Work out the finished part from the listing and answer in its coordinate system (mm). A direction names the side the tool comes from. Give positions to 0.01 mm unless a question says otherwise; leave off trailing zeros. Write each loop counter-clockwise with the first axis right and the second up, starting at its lowest first coordinate (ties: lowest second). Pieces come first, ordered by that corner, then holes.
1) A tool of negligible diameter and unlimited length cuts with its end or side. For faces 1 (the face through (-110.6, -411.4, 382.62)), 2 (the face through (-313.79, -222.74, 380.68)), from which of +Z, -Z, +X, -X, +Y, -Y can it reach the whole face along a straight path? Write none if from no direction.
2) Straight lines are drawn through the part: probe 1 along X at (y, z) = (-526, 378.5); probe 2 along Y at (x, z) = (-32, 381.25); probe 3 along Y at (x, z) = (-26, 379.5). For each, find the intervals that lie inside material, in ascending order.
3) Find section B-B (z = 379). Count the separate pieces of the cut face and the enclosed holes in it, plus the area to 3 significant figures.
4) Determine the mould class of faces 3 (the face through (-44.44, -546.24, 380.68)), 4 (the face through (-108, -396, 384.62)) for opening direction X: pulls with the +X half, pulls with the -X half, needs draft (parallel to the pull), parting line crosses it, or undercut.
5) Given pin 1 Ø4.5 at (x, y) = (-269.36, -538.87) entering from -Z, flat-ended and moving along its own axis, determine where the tip first touches the part or whether it passes through.
6) Find section A-A (x = -112.5). Determine the outline of the cut face in (y, z).
```python
from build123d import *

# Parameters (mm, degrees)
SKETCH1_R           = 6
SKETCH1_R_2         = 4.5
SKETCH1_R_3         = 6.5
SKETCH1_R_4         = 3.735
SKETCH1_W           = 48
SKETCH1_H           = 20
SKETCH1_W_2         = 49
BOSS_EXTRUDE1_DEPTH = 8
SKETCH2_R           = 2.5
CUT_EXTRUDE1_DEPTH  = 10
CUT_EXTRUDE2_DEPTH  = 2


with BuildPart() as part:
    # Sketch1 → Boss-Extrude1 (new body)
    with BuildSketch(Plane(origin=(0, 0, 384.620141885), x_dir=(-1, 0, 0), z_dir=(0, 0, -1))):
        with BuildLine():
            Line((-108.789156386, -197.798939869), (-108.789156386, -599.798939869))
            ThreePointArc((-108.789156386, -599.798939869), (-107.617583511, -602.627366994), (-104.789156386, -603.798939869))
            Line((-104.789156386, -603.798939869), (327.210843614, -603.798939869))
            ThreePointArc((327.210843614, -603.798939869), (330.039270738, -602.627366994), (331.210843614, -599.798939869))
            Line((331.210843614, -599.798939869), (331.210843614, -197.798939869))
            ThreePointArc((331.210843614, -197.798939869), (330.039270738, -194.970512745), (327.210843614, -193.798939869))
            Line((327.210843614, -193.798939869), (-104.789156386, -193.798939869))
            ThreePointArc((-104.789156386, -193.798939869), (-107.617583511, -194.970512745), (-108.789156386, -197.798939869))
        make_face()
        with Locations((-95.789156386, -206.798939869)):
            Circle(SKETCH1_R, mode=Mode.SUBTRACT)
        with Locations((-95.789156386, -226.798939869)):
            Circle(SKETCH1_R, mode=Mode.SUBTRACT)
        with Locations((146.210843614, -209.798939869)):
            Circle(SKETCH1_R_2, mode=Mode.SUBTRACT)
        with Locations((76.210843614, -209.798939869)):
            Circle(SKETCH1_R_2, mode=Mode.SUBTRACT)
        with Locations((318.210843614, -206.798939869)):
            Circle(SKETCH1_R, mode=Mode.SUBTRACT)
        with Locations((318.210843614, -226.798939869)):
            Circle(SKETCH1_R, mode=Mode.SUBTRACT)
        with Locations((-95.789156386, -443.798939869)):
            Circle(SKETCH1_R, mode=Mode.SUBTRACT)
        with Locations((-95.789156386, -463.798939869)):
            Circle(SKETCH1_R, mode=Mode.SUBTRACT)
        with Locations((318.210843614, -443.798939869)):
            Circle(SKETCH1_R, mode=Mode.SUBTRACT)
        with Locations((318.210843614, -463.798939869)):
            Circle(SKETCH1_R, mode=Mode.SUBTRACT)
        with Locations((71.210843614, -480.298939869)):
            Circle(SKETCH1_R, mode=Mode.SUBTRACT)
        with Locations((151.210843614, -480.298939869)):
            Circle(SKETCH1_R, mode=Mode.SUBTRACT)
        with Locations((21.210843614, -551.298939869)):
            Circle(SKETCH1_R, mode=Mode.SUBTRACT)
        with Locations((41.210843614, -551.298939869)):
            Circle(SKETCH1_R, mode=Mode.SUBTRACT)
        with Locations((111.210843614, -560.298939869)):
            Circle(SKETCH1_R_3, mode=Mode.SUBTRACT)
        with Locations((181.210843614, -551.298939869)):
            Circle(SKETCH1_R, mode=Mode.SUBTRACT)
        with Locations((269.360529317, -538.868166644)):
            Circle(SKETCH1_R_4, mode=Mode.SUBTRACT)
        with Locations((201.210843614, -551.298939869)):
            Circle(SKETCH1_R, mode=Mode.SUBTRACT)
        with Locations((31.210843614, -520.298939869)):
            Rectangle(SKETCH1_W, SKETCH1_H, mode=Mode.SUBTRACT)
        with Locations((191.210843614, -520.298939869)):
            Rectangle(SKETCH1_W_2, SKETCH1_H, mode=Mode.SUBTRACT)
    extrude(amount=BOSS_EXTRUDE1_DEPTH)

    # Sketch2 → Cut-Extrude1 (cut)
    with BuildSketch(Plane(origin=(0, 0, 384.620141885), x_dir=(-1, 0, 0), z_dir=(0, 0, -1))):
        with Locations((-94.688937296, -240.632664804)):
            Circle(SKETCH2_R)
        with Locations((317.195009352, -240.632664804)):
            Circle(SKETCH2_R)
    extrude(amount=CUT_EXTRUDE1_DEPTH, mode=Mode.SUBTRACT)

    # Sketch3 → Cut-Extrude2 (cut)
    with BuildSketch(Plane.XY.offset(384.620141885)):
        Polygon((92.937374464, -238.848840921), (96.278253898, -242.562450475), (-253.706289527, -538.668659239), (-256.416648587, -561.465752351), (-261.936974764, -560.809437707), (-258.651893581, -536.026212702), (-319.695009352, -240.632664804), (-314.695009352, -240.632664804), (-254.069511981, -532.152999711), align=None)
    extrude(amount=-CUT_EXTRUDE2_DEPTH, mode=Mode.SUBTRACT)


solid = part.part
```
Results:
1. face 1: +Z
1. face 2: +Z, -Z
2. probe 1: x = -331.21 to -215.71, -166.71 to -55.21, -7.21 to 108.79
2. probe 2: y = -603.8 to -530.3, -510.3 to -193.8
2. probe 3: y = -603.8 to -554.91, -547.68 to -530.3, -510.3 to -193.8
3. separate pieces: 1
3. enclosed holes: 22
3. area: 177,000 mm2
4. face 3: undercut
4. face 4: needs draft
5. pin 1: passes through
6. outline: (-603.8, 376.62) - (-566.67, 376.62) - (-566.67, 384.62) - (-603.8, 384.62) - close; (-553.93, 376.62) - (-193.8, 376.62) - (-193.8, 384.62) - (-412.49, 384.62) - (-412.49, 382.62) - (-419.2, 382.62) - (-419.2, 384.62) - (-553.93, 384.62) - close
